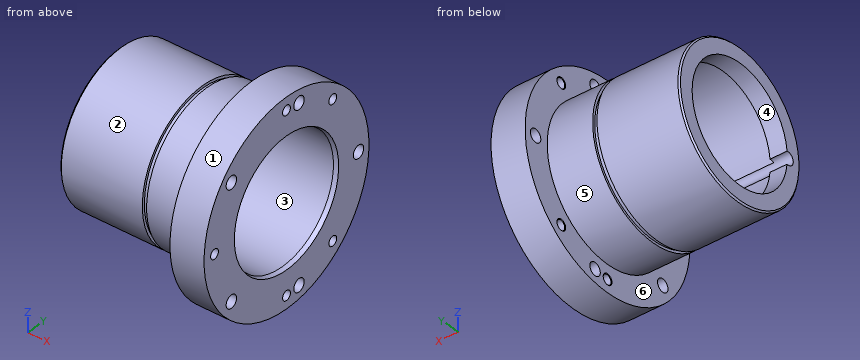
```python
from build123d import *

# Parameters (mm, degrees)
CHAMFER1_SIZE      = 1.5875
CHAMFER2_SIZE      = 4.7752
CHAMFER2_SIZE2     = 1.279510984
SKETCH2_R          = 7.112
CUT_EXTRUDE1_DEPTH = 163.7284
SKETCH3_R          = 7.14375
CUT_EXTRUDE2_DEPTH = 218.327643362
CIRPATTERN1_COUNT  = 18
CIRPATTERN2_COUNT  = 36


with BuildPart() as part:
    # Sketch1 → Revolve1 (revolve)
    with BuildSketch(Plane.XY, mode=Mode.PRIVATE) as revolve1_sk:
        Polygon((0, 65.0875), (0, 82.54238), (92.1004, 82.54238), (92.1004, 79.7052), (96.9264, 79.7052), (96.9264, 82.54238), (147.7264, 82.54238), (147.7264, 112.7125), (185.8264, 112.7125), (185.8264, 70.04685), (19.05, 70.04685), (19.05, 65.0875), align=None)
    revolve(revolve1_sk.sketch.rotate(Axis((0, 0, 0), (1, 0, 0)), 90), axis=Axis((0, 0, 0), (1, 0, 0)))

    # Chamfer1
    chamfer1_edges = [part.edges().sort_by_distance(p)[0] for p in [
        (0, 0, -82.54238),
    ]]
    chamfer(chamfer1_edges, length=CHAMFER1_SIZE)

    # Chamfer2
    chamfer2_edges = [part.edges().sort_by_distance(p)[0] for p in [
        (185.8264, 0, -70.04685),
    ]]
    chamfer2_side = [part.faces().sort_by_distance(p)[0] for p in [
        (102.4382, 0, -70.04685),
    ]]
    chamfer(chamfer2_edges, length=CHAMFER2_SIZE, length2=CHAMFER2_SIZE2, reference=chamfer2_side[0])

    # Sketch2 → Cut-Extrude1 (cut)
    with BuildSketch(Plane.ZY):
        with Locations((0, -66.10985)):
            Circle(SKETCH2_R)
    extrude(amount=-CUT_EXTRUDE1_DEPTH, mode=Mode.SUBTRACT)

    # Sketch3 → Cut-Extrude2 (cut, through all)
    with BuildSketch(Plane.ZY.offset(-147.7264)):
        with Locations((0, 98.425)):
            Circle(SKETCH3_R)
    cut_extrude2 = extrude(amount=-CUT_EXTRUDE2_DEPTH, mode=Mode.SUBTRACT)

    # CirPattern1: Cut-Extrude2 ×18 about axis, 13 skipped
    cirpattern1_axis = Axis((147.7264, 0, 0), (-1, 0, 0))
    add([cut_extrude2.rotate(cirpattern1_axis, i * 360 / CIRPATTERN1_COUNT) for i in range(1, CIRPATTERN1_COUNT) if i not in (1, 2, 3, 5, 6, 8, 9, 10, 12, 13, 15, 16, 17)], mode=Mode.SUBTRACT)

    # Sketch5 → Tap Drill for 1/2-13 Tap1 (revolve, cut)
    with BuildSketch(Plane(origin=(147.7264, -98.425, 0), x_dir=(0, 0, 1), z_dir=(0, 1, 0))):
        Polygon((0, 0), (0, 41.319489309), (5.35813, 38.1), (5.35813, 0.532828266), (5.99313, 0), align=None)
    tap_drill_for_1_2_13_tap1 = revolve(axis=Axis((141.3764, -98.425, 0), (1, 0, 0)), mode=Mode.SUBTRACT)

    # CirPattern2: Tap Drill for 1/2-13 Tap1 ×36 about axis, 31 skipped
    cirpattern2_axis = Axis((147.7264, 0, 0), (-1, 0, 0))
    add([tap_drill_for_1_2_13_tap1.rotate(cirpattern2_axis, i * 360 / CIRPATTERN2_COUNT) for i in range(1, CIRPATTERN2_COUNT) if i not in (1, 2, 3, 4, 5, 6, 7, 8, 10, 11, 12, 14, 15, 16, 17, 18, 19, 20, 21, 22, 24, 25, 26, 28, 29, 30, 31, 32, 33, 34, 35)], mode=Mode.SUBTRACT)


solid = part.part
```
Model file for the job. Use its own axes, mm. Face numbers are marked on the shaded views. A direction names the side the tool comes from. Give positions to 0.01 mm unless a question says otherwise; leave off trailing zeros. Order: outer loops, then holes, each group sorted by start corner. A loop starts at its lowest first (then second) coordinate and runs counter-clockwise, first axis right, second up.
1) Saw through at A-A, the plane x = 23. Write the cut outline in (y, z).
2) Wall check: probe 1 along Z at (x, y) = (168.5, 22); probe 2 along X at (y, z) = (-87.5, 4); probe 3 along Z at (x, y) = (124, 39.5). Give the ranges that are in metal, low to high.
3) 3-axis set-ups, long thin cutter, end or side, ignore diameter. For the marked faces 1 and 2: which of +Z, -Z, +X, -X, +Y, -Y reach the whole face in a straight line?
4) Pin check, flat tips, straight feed: pin 1 (6.5 mm diameter, centred on y = 63.27, z = 75.4, fed in from +X); pin 2 (18.5 mm diameter, centred on y = -75.4, z = -63.27, fed in from -X); pin 3 (23 mm diameter, centred on y = 98.425, z = 0, fed in from +X); pin 4 (6 mm diameter, centred on x = 156, y = -26, fed in from -Z). Stop position of each tip, or through.
5) Mould opens along Y. For the marked faces 3, 4, 5 and 6 say: +Y half, -Y half, draft (parallel to the pull), parting line (faces both ways), or undercut.
6) Saw through at B-B, the plane y = 0. Count the separate pieces of the cut face and the enclosed holes in it, then the cut area to 3 significant figures.
Computed:
1. outline: circle Ø165.08 at (0, 0); hole (-69.78, -6.09) arc R70.05 ccw (long way) to (-69.78, 6.09) arc R7.11 ccw to start
2. probe 1: z = -110.54 to -102.12, -91.74 to -66.5, 66.5 to 91.74, 102.12 to 110.54
2. probe 2: x = 147.73 to 185.83
2. probe 3: z = -72.48 to -57.85, 57.85 to 72.48
3. face 1: +X, -X
3. face 2: -X
4. pin 1: passes through
4. pin 2: stops at x = 147.73
4. pin 3: stops at x = 185.83
4. pin 4: stops at z = -110.34
5. face 3: undercut
5. face 4: undercut
5. face 5: parting line
5. face 6: draft
6. separate pieces: 4
6. enclosed holes: 0
6. area: 6,280 mm2
